Can you work these out from the model? Positions are in its coordinate system, mm. A direction names the side the tool comes from. Round coordinates to 2 decimals unless told otherwise and drop trailing zeros. Order: outer loops, then holes, each group sorted by start corner. A loop starts at its lowest first (then second) coordinate and runs counter-clockwise, first axis right, second up. Notation, with made-up numbers: (-4, -5.5) - (55, -5.5) arc R22 cw to (55, 25.5) - close; hole circle Ø6 at (67.5, -14.5). An arc over 180 degrees is marked (long way). Write item = value, one per line.
from build123d import *

# Parameters (mm, degrees)
F1_DEPTH = 2
F0_R     = 3
F0_R_2   = 1.5
F2_DEPTH = 5
F3_DEPTH = 5


with BuildPart() as f1:
    # F0 (on Top) → F1 (new body)
    with BuildSketch(Plane.XY):
        with BuildLine():
            Line((-5.4919344625, -24.5), (5.7497143832, -24.5))
            ThreePointArc((5.7497143832, -24.5), (8.5080655375, -22.6796181202), (11.2664166918, -24.5))
            Line((11.2664166918, -24.5), (22.5080655375, -24.5))
            ThreePointArc((22.5080655375, -24.5), (23.2151723187, -24.2071067812), (23.5080655375, -23.5))
            Line((23.5080655375, -23.5), (23.5080655375, -20))
            ThreePointArc((23.5080655375, -20), (22.9222790999, -21.4142135624), (21.5080655375, -22))
            Line((21.5080655375, -22), (-4.4919344625, -22))
            ThreePointArc((-4.4919344625, -22), (-5.9061480249, -21.4142135624), (-6.4919344625, -20))
            Line((-6.4919344625, -20), (-6.4919344625, -23.5))
            ThreePointArc((-6.4919344625, -23.5), (-6.1990412437, -24.2071067812), (-5.4919344625, -24.5))
        make_face()
    extrude(amount=F1_DEPTH)

    # F0 (on Top) → F2 (join)
    with BuildSketch(Plane.XY):
        with BuildLine():
            Line((23.0080655375, 18), (-7.9919344625, 18))
            ThreePointArc((-7.9919344625, 18), (-9.4061480249, 17.4142135624), (-9.9919344625, 16))
            Line((-9.9919344625, 16), (-9.9919344625, 13.0157731473))
            Line((-9.9919344625, 13.0157731473), (-9.9919344625, -25))
            ThreePointArc((-9.9919344625, -25), (-9.4061480249, -26.4142135624), (-7.9919344625, -27))
            Line((-7.9919344625, -27), (5.8142593657, -27))
            ThreePointArc((5.8142593657, -27), (5.5090648911, -25.7570462979), (5.7497143832, -24.5))
            Line((5.7497143832, -24.5), (-5.4919344625, -24.5))
            ThreePointArc((-5.4919344625, -24.5), (-6.1990412437, -24.2071067812), (-6.4919344625, -23.5))
            Line((-6.4919344625, -23.5), (-6.4919344625, -20))
            Line((-6.4919344625, -20), (-6.4919344625, -2))
            ThreePointArc((-6.4919344625, -2), (-5.9061480249, -0.5857864376), (-4.4919344625, 0))
            Line((-4.4919344625, 0), (-3.4919344625, 0))
            ThreePointArc((-3.4919344625, 0), (-2.0777209001, 0.5857864376), (-1.4919344625, 2))
            Line((-1.4919344625, 2), (-1.4919344625, 3.6054256072))
            ThreePointArc((-1.4919344625, 3.6054256072), (-1.1324864177, 4.7493614806), (-0.1833451802, 5.4821118409))
            Line((-0.1833451802, 5.4821118409), (14.8166548198, 11.0084276303))
            ThreePointArc((14.8166548198, 11.0084276303), (16.6520014109, 10.7722933519), (17.5080655375, 9.1317413967))
            Line((17.5080655375, 9.1317413967), (17.5080655375, -1))
            ThreePointArc((17.5080655375, -1), (18.0938519751, -2.4142135624), (19.5080655375, -3))
            Line((19.5080655375, -3), (21.5080655375, -3))
            ThreePointArc((21.5080655375, -3), (22.9222790999, -3.5857864376), (23.5080655375, -5))
            Line((23.5080655375, -5), (23.5080655375, -20))
            Line((23.5080655375, -20), (23.5080655375, -23.5))
            ThreePointArc((23.5080655375, -23.5), (23.2151723187, -24.2071067812), (22.5080655375, -24.5))
            Line((22.5080655375, -24.5), (11.2664166918, -24.5))
            ThreePointArc((11.2664166918, -24.5), (11.4470324872, -25.0775605909), (11.5080655375, -25.6796181202))
            ThreePointArc((11.5080655375, -25.6796181202), (11.4305147257, -26.357328045), (11.2018717093, -27))
            Line((11.2018717093, -27), (25.0080655375, -27))
            ThreePointArc((25.0080655375, -27), (26.4222790999, -26.4142135624), (27.0080655375, -25))
            Line((27.0080655375, -25), (27.0080655375, -1))
            ThreePointArc((27.0080655375, -1), (26.7151723187, -0.2928932188), (26.0080655375, 0))
            ThreePointArc((26.0080655375, 0), (25.3009587563, 0.2928932188), (25.0080655375, 1))
            Line((25.0080655375, 1), (25.0080655375, 13.0157731473))
            Line((25.0080655375, 13.0157731473), (25.0080655375, 16))
            ThreePointArc((25.0080655375, 16), (24.4222790999, 17.4142135624), (23.0080655375, 18))
        make_face()
        with BuildLine():
            ThreePointArc((-3.9919344625, 13.0157731473), (-6.9919344625, 10.0157731473), (-9.9919344625, 13.0157731473))
            ThreePointArc((-9.9919344625, 13.0157731473), (-6.9919344625, 16.0157731473), (-3.9919344625, 13.0157731473))
        make_face(mode=Mode.SUBTRACT)
        with Locations((22.0080655375, 13.0157731473)):
            Circle(F0_R, mode=Mode.SUBTRACT)
        with BuildLine():
            ThreePointArc((-3.9919344625, 13.0157731473), (-6.9919344625, 16.0157731473), (-9.9919344625, 13.0157731473))
            ThreePointArc((-9.9919344625, 13.0157731473), (-6.9919344625, 10.0157731473), (-3.9919344625, 13.0157731473))
        make_face()
        with Locations((-6.9919344625, 13.0157731473)):
            Circle(F0_R_2, mode=Mode.SUBTRACT)
        with Locations((22.0080655375, 13.0157731473)):
            Circle(F0_R)
        with Locations((22.0080655375, 13.0157731473)):
            Circle(F0_R_2, mode=Mode.SUBTRACT)
        with BuildLine():
            Line((7.7963129882, -27), (5.8142593657, -27))
            ThreePointArc((5.8142593657, -27), (8.5080655375, -28.6796181202), (11.2018717093, -27))
            Line((11.2018717093, -27), (9.2198180868, -27))
            ThreePointArc((9.2198180868, -27), (8.5080655375, -27.1796181202), (7.7963129882, -27))
        make_face()
        with BuildLine():
            ThreePointArc((5.7497143832, -24.5), (5.5090648911, -25.7570462979), (5.8142593657, -27))
            Line((5.8142593657, -27), (7.7963129882, -27))
            ThreePointArc((7.7963129882, -27), (7.0135717951, -25.8080254948), (7.5815121982, -24.5))
            Line((7.5815121982, -24.5), (5.7497143832, -24.5))
        make_face()
        with BuildLine():
            Line((9.2198180868, -27), (11.2018717093, -27))
            ThreePointArc((11.2018717093, -27), (11.4305147257, -26.357328045), (11.5080655375, -25.6796181202))
            ThreePointArc((11.5080655375, -25.6796181202), (11.4470324872, -25.0775605909), (11.2664166918, -24.5))
            Line((11.2664166918, -24.5), (9.4346188768, -24.5))
            ThreePointArc((9.4346188768, -24.5), (9.857107792, -25.0238094625), (10.0080655375, -25.6796181202))
            ThreePointArc((10.0080655375, -25.6796181202), (9.7960152306, -26.4485040597), (9.2198180868, -27))
        make_face()
    extrude(amount=F2_DEPTH)

    # F0 (on Top) → F3 (join)
    with BuildSketch(Plane.XY):
        with BuildLine():
            ThreePointArc((11.2664166918, -24.5), (8.5080655375, -22.6796181202), (5.7497143832, -24.5))
            Line((5.7497143832, -24.5), (7.5815121982, -24.5))
            ThreePointArc((7.5815121982, -24.5), (8.5080655375, -24.1796181202), (9.4346188768, -24.5))
            Line((9.4346188768, -24.5), (11.2664166918, -24.5))
        make_face()
    extrude(amount=F3_DEPTH)


solid = f1.part
(1) If I drill on line 1 (Y direction, x = 22.5, z = 4.85); line 2 (X direction, y = 13, z = 1.1); line 3 (Y direction, x = 7.5, z = 1.65), over which ranges is the centre line in solid material (lowest first)? Write a range as from..to.
Computed:
line_1 = -27..-24.5, -3.26..11.6, 14.43..18
line_2 = -9.99..-8.49, -5.49..20.51, 23.51..25.01
line_3 = -28.51..-26.79, -24.57..-22, 8.31..18
(2) If we section it at B-B (x = 12): Write out the boundary of the cut face in (y, z).
Computed:
outline = (-27, 0) - (-22, 0) - (-22, 2) - (-24.5, 2) - (-24.5, 5) - (-27, 5) - close; (9.97, 0) - (18, 0) - (18, 5) - (9.97, 5) - close
(3) If we section it at A-A (y = -9): Write out the boundary of the cut face in (x, z), plus the area to 3 significant figures.
Computed:
outline = (-9.99, 0) - (-6.49, 0) - (-6.49, 5) - (-9.99, 5) - close; (23.51, 0) - (27.01, 0) - (27.01, 5) - (23.51, 5) - close
area = 35.0 mm^2
(4) If we section it at D-D (x = 3): Write out the boundary of the cut face in (y, z), plus the area to 3 significant figures.
Computed:
outline = (-27, 0) - (-22, 0) - (-22, 2) - (-24.5, 2) - (-24.5, 5) - (-27, 5) - close; (6.65, 0) - (18, 0) - (18, 5) - (6.65, 5) - close
area = 74.2 mm^2
(5) On a 3-axis mill with a long thin cutter (end or side, diameter ignored), from which of +Z, -Z, +X, -X, +Y, -Y can I reach the whole of each face in a straight line? I mean faces 1 (the face through (22.907, -3.57, 2.465)), 2 (the face through (18, -27, 2)), 3 (the face through (25.008, 8, 2)), 4 (the face through (17, -24.5, 3)), 5 (the face through (-1, -27, 2)). Say none if no direction works.
Computed:
face_1 = +Z, -Z
face_2 = +Z, -Z, +X, -Y
face_3 = +Z, -Z, +X, +Y
face_4 = +Z
face_5 = +Z, -Z, -X, -Y
(6) Will these pins go through, and if not, where does the flat tip stop? P1, Ø2, axis at x = 13, y = -21.5, coming from the +Z side; P2, Ø12, axis at x = 6, y = -8, coming from the -Z side; P3, Ø2, axis at x = 20.5, z = 1.5, coming from the -Y side; P4, Ø1.3, axis at y = 2.5, z = 3.5, coming from the +X side.
Computed:
P1 = 2
P2 = through
P3 = -27
P4 = 25.01
(7) If we section it at C-C (y = 7.5): Write out the boundary of the cut face in (x, z), plus the area to 3 significant figures.
Computed:
outline = (-9.99, 0) - (5.29, 0) - (5.29, 5) - (-9.99, 5) - close; (17.51, 0) - (25.01, 0) - (25.01, 5) - (17.51, 5) - close
area = 114 mm^2
